```python
from build123d import *

# Parameters (mm, degrees)
CROQUIS1_R              = 5
SALIENTE_EXTRUIR1_DEPTH = 15
CROQUIS2_W              = 130
CROQUIS2_H              = 5
CORTAR_EXTRUIR1_DEPTH   = 138.295302177


with BuildPart() as part:
    # Croquis1 → Saliente-Extruir1 (new body)
    with BuildSketch(Plane.XY):
        with BuildLine():
            Line((0, 10), (125, 10))
            ThreePointArc((125, 10), (135, 0), (125, -10))
            Line((125, -10), (0, -10))
            ThreePointArc((0, -10), (-10, 0), (0, 10))
        make_face()
        Circle(CROQUIS1_R, mode=Mode.SUBTRACT)
    extrude(amount=SALIENTE_EXTRUIR1_DEPTH)

    # Croquis2 → Cortar-Extruir1 (cut, through all)
    with BuildSketch(Plane(origin=(0, 10, 0), x_dir=(1, 0, 0), z_dir=(0, 1, 0))):
        with Locations((55, -7.5)):
            Rectangle(CROQUIS2_W, CROQUIS2_H)
    extrude(amount=-CORTAR_EXTRUIR1_DEPTH, mode=Mode.SUBTRACT)


solid = part.part
```
Check sheet for the modelled part. Datum: model origin and axes. Units: mm. A direction names the side the tool comes from. Give positions to 0.01 mm unless a question says otherwise; leave off trailing zeros. Write each loop counter-clockwise with the first axis right and the second up, starting at its lowest first coordinate (ties: lowest second). Pieces come first, ordered by that corner, then holes.
Item 1: Cross-section at D-D (y = 8.5). Enter the section's corners in (x, z).
Item 2: Cross-section at C-C (z = 1.75). Enter the section's corners in (x, y), and give its area (3 significant figures).
Item 3: Gauge pin test, flat ends, axial feed: pin 1 (1 mm diameter, centred on y = -5.5, z = 2.5, fed in from -X); pin 2 (1.5 mm diameter, centred on y = -3, z = 6.5, fed in from -X); pin 3 (2 mm diameter, centred on y = -5, z = 5, fed in from -X). Record the tip position at first contact, or that the pin passes through.
Item 4: Scan lines: L1, parallel to Z at x = 44, y = 9; L2, parallel to Y at x = 0, z = 13; L3, parallel to X at y = 0, z = 13.85. Record each from-to range of solid material in increasing order.
Item 5: Cross-section at A-A (x = 54). Enter the section's corners in (y, z).
Item 6: Access from +Z, -Z, +X, -X, +Y, -Y to the whole of each face (thin tool, end or side, straight path). Record for faces 1 (the face through (135, 0, 7)), 2 (the face through (120, 0, 8)).
Item 7: Cross-section at B-B (y = 0). Enter the section's corners in (x, z).
Item 8: Draft check along Z on faces 3 (the face through (64, 0, 0)), 4 (the face through (54, 0, 10)), 5 (the face through (54, 0, 5)), 6 (the face through (-10, 0, 12)). Enter one of: released by +Z, released by -Z, zero draft, split by the parting line, or undercut.
Report:
1. outline: (-5.27, 0) - (130.27, 0) - (130.27, 15) - (-5.27, 15) - (-5.27, 10) - (120, 10) - (120, 5) - (-5.27, 5) - close
2. outline: (0, -10) - (125, -10) arc R10 ccw to (125, 10) - (0, 10) arc R10 ccw to start; hole circle Ø10 at (0, 0)
2. area: 2,740 mm2
3. pin 1: stops at x = -8.66
3. pin 2: stops at x = 120
3. pin 3: stops at x = -9.17
4. L1: z = 0 to 5, 10 to 15
4. L2: y = -10 to -5, 5 to 10
4. L3: x = -10 to -5, 5 to 135
5. outline: (-10, 0) - (10, 0) - (10, 5) - (-10, 5) - close; (-10, 10) - (10, 10) - (10, 15) - (-10, 15) - close
6. face 1: +Z, -Z, +X
6. face 2: -X, +Y, -Y
7. outline: (-10, 0) - (-5, 0) - (-5, 5) - (-10, 5) - close; (-10, 10) - (-5, 10) - (-5, 15) - (-10, 15) - close; (5, 0) - (135, 0) - (135, 15) - (5, 15) - (5, 10) - (120, 10) - (120, 5) - (5, 5) - close
8. face 3: released by -Z
8. face 4: undercut
8. face 5: undercut
8. face 6: zero draft
